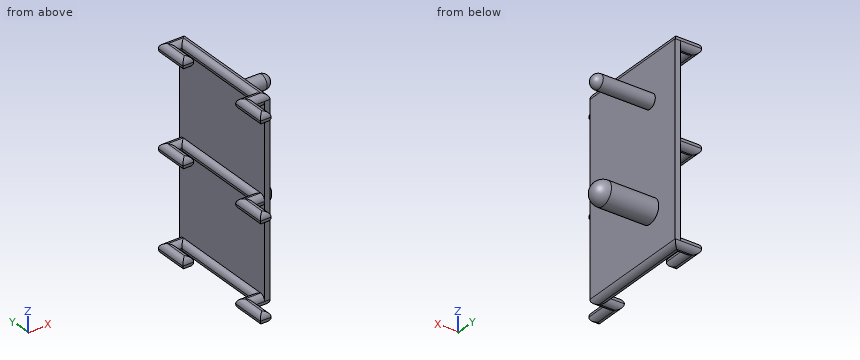
from build123d import *
from OCP.BRepFilletAPI import BRepFilletAPI_MakeFillet

# Parameters (mm, degrees)
EXTRU_MINCE1_DEPTH           = 2.3
CONG_1_R                     = 2.3
ESQUISSE2_W                  = 80
ESQUISSE2_H                  = 49.6
BOSS_EXTRU_1_DEPTH           = 2.3
R_P_TITION_START             = 77.7
R_P_TITION_LIN_AIRE1_DEPTH   = 4.6
R_P_TITION_START_2           = 37.7
R_P_TITION_LIN_AIRE1_2_DEPTH = 4.6
CONG_2_R                     = 2.3
ESQUISSE3_R                  = 3
ESQUISSE3_R_2                = 5
BOSS_EXTRU_2_DEPTH           = 25
CONG_5_R1                    = 3
CONG_5_R2                    = 5


# Read off the part's stored shape, not the designer's step: Répétition linéaire1
with BuildPart() as part:
    # Esquisse1 → Extru.-Mince1 (new, symmetric)
    with BuildSketch(Plane.XY):
        Polygon((-4.3, -57), (-4.3, -47.3), (2.3, -47.3), (2.3, 2.3), (-8.9, 2.3), (-8.9, -12), (-4.3, -12), (-4.3, -2.3), (-2.3, -2.3), (-2.3, -42.7), (-8.9, -42.7), (-8.9, -57), align=None)
    extrude(amount=EXTRU_MINCE1_DEPTH, both=True)

    # Congé1
    cong_1_edges = [part.edges().sort_by_distance(p)[0] for p in [
        (-6.6, -57, -2.3),
        (-4.3, -52.15, -2.3),
        (-1, -47.3, -2.3),
        (2.3, -22.5, -2.3),
        (-3.3, 2.3, -2.3),
        (-8.9, -4.85, -2.3),
        (-6.6, -12, -2.3),
        (-4.3, -7.15, -2.3),
        (-3.3, -2.3, -2.3),
        (-2.3, -22.5, -2.3),
        (-5.6, -42.7, -2.3),
        (-8.9, -49.85, -2.3),
        (-5.6, -42.7, 2.3),
        (-2.3, -22.5, 2.3),
        (-3.3, -2.3, 2.3),
        (-4.3, -7.15, 2.3),
        (-6.6, -12, 2.3),
        (-8.9, -4.85, 2.3),
        (-3.3, 2.3, 2.3),
        (2.3, -22.5, 2.3),
        (-1, -47.3, 2.3),
        (-4.3, -52.15, 2.3),
        (-6.6, -57, 2.3),
        (-8.9, -49.85, 2.3),
    ]]
    fillet(cong_1_edges, radius=CONG_1_R - 0.0001)  # a hair under: the kernel refuses the full size

    # Esquisse2 → Boss.-Extru.1 (add)
    with BuildSketch(Plane(origin=(0, 0, 0), x_dir=(0, 0, -1), z_dir=(1, 0, 0))):
        with Locations((-40, -22.5)):
            Rectangle(ESQUISSE2_W, ESQUISSE2_H)
    extrude(amount=BOSS_EXTRU_1_DEPTH)

    # Répétition linéaire1 outline → Répétition linéaire1 (add)
    with BuildSketch(Plane.XY.offset(R_P_TITION_START)):
        Polygon((-8.9, 2.3), (-8.9, -12), (-4.3, -12), (-4.3, -2.3), (-2.3, -2.3), (-2.3, -42.7), (-8.9, -42.7), (-8.9, -57), (-4.3, -57), (-4.3, -47.3), (2.3, -47.3), (2.3, 2.3), align=None)
    extrude(amount=R_P_TITION_LIN_AIRE1_DEPTH)

    # R_p_tition lin_aire1 2 outline → R_p_tition lin_aire1 2 (add)
    with BuildSketch(Plane.XY.offset(R_P_TITION_START_2)):
        Polygon((0, 2.3), (-8.9, 2.3), (-8.9, -12), (-4.3, -12), (-4.3, -2.3), (-2.3, -2.3), (-2.3, -42.7), (-8.9, -42.7), (-8.9, -57), (-4.3, -57), (-4.3, -47.3), (0, -47.3), align=None)
    extrude(amount=R_P_TITION_LIN_AIRE1_2_DEPTH)

    # Congé2
    cong_2_edges = [part.edges().sort_by_distance(p)[0] for p in [
        (2.3, -22.5, 82.3),
        (-1, -47.3, 82.3),
        (-3.3, 2.3, 82.3),
        (-4.45, 2.3, 77.7),
        (-2.15, -47.3, 77.7),
        (-4.3, -52.15, 77.7),
        (-6.6, -57, 77.7),
        (-6.6, -12, 77.7),
        (-8.9, -4.85, 77.7),
        (-8.9, -49.85, 77.7),
        (-6.6, -57, 82.3),
        (-4.3, -52.15, 82.3),
        (-8.9, -4.85, 82.3),
        (-6.6, -12, 82.3),
        (-4.3, -7.15, 77.7),
        (-3.3, -2.3, 77.7),
        (-2.3, -22.5, 77.7),
        (-5.6, -42.7, 77.7),
        (-8.9, -49.85, 82.3),
        (-4.3, -7.15, 82.3),
        (-3.3, -2.3, 82.3),
        (-2.3, -22.5, 82.3),
        (-5.6, -42.7, 82.3),
        (-2.15, -47.3, 42.3),
        (-4.45, 2.3, 42.3),
        (-4.3, -7.15, 42.3),
        (-3.3, -2.3, 42.3),
        (-2.3, -22.5, 42.3),
        (-5.6, -42.7, 42.3),
        (-8.9, -49.85, 42.3),
        (-4.45, 2.3, 37.7),
        (-2.15, -47.3, 37.7),
        (-4.3, -52.15, 37.7),
        (-6.6, -57, 37.7),
        (-6.6, -12, 37.7),
        (-8.9, -4.85, 37.7),
        (-8.9, -49.85, 37.7),
        (-6.6, -57, 42.3),
        (-4.3, -52.15, 42.3),
        (-8.9, -4.85, 42.3),
        (-6.6, -12, 42.3),
        (-4.3, -7.15, 37.7),
        (-3.3, -2.3, 37.7),
        (-2.3, -22.5, 37.7),
        (-5.6, -42.7, 37.7),
    ]]
    fillet(cong_2_edges, radius=CONG_2_R - 0.0001)  # a hair under: the kernel refuses the full size

    # Esquisse3 → Boss.-Extru.2 (add)
    with BuildSketch(Plane(origin=(2.3, 0, 0), x_dir=(0, 0, -1), z_dir=(1, 0, 0))):
        with Locations((-62, -12.3)):
            Circle(ESQUISSE3_R)
        with Locations((-18, -12.3)):
            Circle(ESQUISSE3_R_2)
    extrude(amount=BOSS_EXTRU_2_DEPTH)

    # Congé5: one fillet with a radius per group of edges: ONE call of the kernel's fillet builder (fillet() takes one radius for all edges)
    cong_5_edges_1 = [part.edges().sort_by_distance(p)[0] for p in [
        (27.3, -12.3, 65),
    ]]
    cong_5_edges_2 = [part.edges().sort_by_distance(p)[0] for p in [
        (27.3, -12.3, 23),
    ]]
    cong_5 = BRepFilletAPI_MakeFillet(part.part.solid().wrapped)
    for e in cong_5_edges_1:
        cong_5.Add(CONG_5_R1, e.wrapped)
    for e in cong_5_edges_2:
        cong_5.Add(CONG_5_R2, e.wrapped)
    add(Compound.cast(cong_5.Shape()), mode=Mode.REPLACE)


solid = part.part
Can you work these out from the model? Positions are in its coordinate system, mm. Coordinates: 2 decimals unless noted, no trailing zeros. Loops run counter-clockwise (first coordinate to the right, second up) from the corner with the lowest first, then second, coordinate; pieces in that order, holes last. Notation, with made-up numbers: (51.25, -29) - (108.25, -29) arc R13 cw to (108.25, -24) - close; hole circle Ø3 at (48.25, -12). An arc over 180 degrees is marked (long way). Answer as a JSON object with one key per item and string values. Group by question number.
Item 1: If we section it at D-D (z = 62): List the corners of the cut face in (x, y) for me.
Item 2: If I drill on L1, parallel to X at y = -20, z = 9; L2, parallel to Y at x = 1.5, z = 25.5; L3, parallel to Z at x = -3, y = -44.5, over which ranges is the centre line in solid material (lowest first)? Write a range as from..to.
Item 3: For pin 1 (1.5 mm diameter, centred on y = -25.5, z = 43.5, fed in from -X); pin 2 (3.5 mm diameter, centred on x = -3, y = -21, fed in from -Z); pin 3 (6 mm diameter, centred on x = 6, y = -6, fed in from +Z), each with a flat end and sliding along its axis, tell me the tip position at first contact or that it passes through.
Item 4: If we section it at A-A (z = 18): List the corners of the cut face in (x, y) for me.
Item 5: If we section it at B-B (x = 10.5): List the corners of the cut face in (y, z) for me.
Returned:
{
 "1": {"outline": "(0, -47.3) - (2.3, -47.3) - (2.3, -15.3) - (24.3, -15.3) arc R3 ccw to (24.3, -9.3) - (2.3, -9.3) - (2.3, 2.3) - (0, 2.3) - close"},
 "2": {"L1": "x = 0..2.3", "L2": "y = -47.3..2.3", "L3": "z = -2.25..2.25, 37.75..42.25, 77.75..82.25"},
 "3": {"pin 1": "stops at x = 0", "pin 2": "stops at z = -1.93", "pin 3": "stops at z = 21.76"},
 "4": {"outline": "(0, -47.3) - (2.3, -47.3) - (2.3, -17.3) - (22.3, -17.3) arc R5 ccw to (22.3, -7.3) - (2.3, -7.3) - (2.3, 2.3) - (0, 2.3) - close"},
 "5": {"outline": "circle Ø10 at (-12.3, 18); circle Ø6 at (-12.3, 62)"}
}
